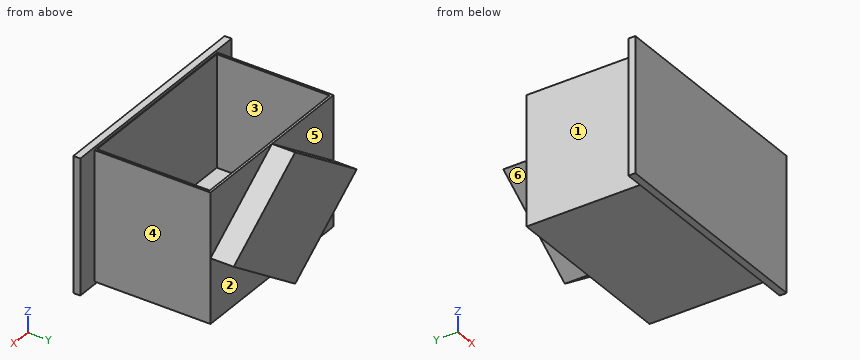
```python
from build123d import *

# Parameters (mm, degrees)
SKETCH_1_W          = 480
SKETCH_1_H          = 290
EXTRUDE_1_DEPTH     = 15
SKETCH_2_W          = 390
SKETCH_2_H          = 178
EXTRUDE_2_DEPTH     = 250
SKETCH_7_W          = 390
SKETCH_7_H          = 250
EXTRUDE_7_DEPTH     = 100
SKETCH_8_W          = 380
SKETCH_8_H          = 243
CUT_EXTRUDE_1_DEPTH = 240
EXTRUDE_8_DEPTH     = 50


with BuildPart() as part:
    # 草图1 → 凸台-拉伸1 (new body)
    with BuildSketch(Plane(origin=(0, 0, 0), x_dir=(1, 0, 0), z_dir=(0, 1, 0))):
        Rectangle(SKETCH_1_W, SKETCH_1_H)
    extrude(amount=-EXTRUDE_1_DEPTH)

    # 草图2 → 凸台-拉伸2 (add)
    with BuildSketch(Plane(origin=(0, 0, 0), x_dir=(1, 0, 0), z_dir=(0, 1, 0))):
        with Locations((0, 50)):
            Rectangle(SKETCH_2_W, SKETCH_2_H)
    extrude(amount=EXTRUDE_2_DEPTH)

    # 草图7 → 凸台-拉伸7 (add)
    with BuildSketch(Plane.XY.offset(39)):
        with Locations((0, 125)):
            Rectangle(SKETCH_7_W, SKETCH_7_H)
    extrude(amount=EXTRUDE_7_DEPTH)

    # 草图8 → 切除-拉伸1 (cut)
    with BuildSketch(Plane.XY.offset(139)):
        with Locations((0, 123.5)):
            Rectangle(SKETCH_8_W, SKETCH_8_H)
    extrude(amount=-CUT_EXTRUDE_1_DEPTH, mode=Mode.SUBTRACT)

    # 草图10 → 凸台-拉伸8 (add)
    with BuildSketch(Plane(origin=(0, 250, 0), x_dir=(1, 0, 0), z_dir=(0, 1, 0))):
        Polygon((0, 139), (-195, 0), (0, -139), (195, 0), align=None)
    extrude(amount=EXTRUDE_8_DEPTH)


solid = part.part
```
Input: part model. Units: mm. Frame: model coordinates. Face numbers are marked on the shaded views. A direction names the side the tool comes from. Coordinates: 2 decimals unless noted, no trailing zeros. Loops run counter-clockwise (first coordinate to the right, second up) from the corner with the lowest first, then second, coordinate; pieces in that order, holes last. Notation, with made-up numbers: M 0.25,77 L 18.25,77 A19 cw 18.25,87 Z; hole C 30.25,-32 d2. An arc over 180 degrees is marked long. One line per item, written item: value.
(1) Reachability of the marked faces 4, 5 and 6 from +Z, -Z, +X, -X, +Y, -Y: full face, straight path, thin tool, end or side. Return the list, or none.
Filled in:
face 4: +Z, -Z, +X, +Y
face 5: +Z, -X, +Y
face 6: -Z, -X, +Y
(2) Section B-B (x = -168.5). Output: boundary loops of the cut face in (y, z), and give its area (3 significant figures).
Filled in:
outline: M -15,-145 L 0,-145 L 0,-139 L 250,-139 L 250,-18.89 L 300,-18.89 L 300,18.89 L 250,18.89 L 250,139 L 245,139 L 245,-101 L 2,-101 L 2,139 L 0,139 L 0,145 L -15,145 Z
area: 17,400 mm^2
(3) Pin query (flat end, axial travel): pin 1 (2 mm diameter, centred on x = 122, z = 81.5, fed in from +Y); pin 2 (10 mm diameter, centred on y = 28, z = -23.5, fed in from +X); pin 3 (1.5 mm diameter, centred on y = 64.5, z = 111, fed in from -X). Return the tip coordinate at first contact, or that it passes through.
Filled in:
pin 1: y = 250
pin 2: x = 195
pin 3: x = -195
(4) Line query: line 1 along X through (y, z) = (45, 15); line 2 along Y through (x, z) = (-120.5, -28.5); line 3 along Y through (x, z) = (175, -40). Output: solid intervals per line, ascending. Write a range as from..to.
Filled in:
line 1: -195..-190, 190..195
line 2: -15..2, 245..300
line 3: -15..2, 245..250
(5) Section C-C (y = 12.5). Output: boundary loops of the cut face in (x, z), and give its area (3 significant figures).
Filled in:
outline: M -195,-139 L 195,-139 L 195,139 L 190,139 L 190,-101 L -190,-101 L -190,139 L -195,139 Z
area: 17,200 mm^2
(6) Section D-D (z = -110.5). Output: boundary loops of the cut face in (x, y), and give its area (3 significant figures).
Filled in:
outline: M -240,-15 L 240,-15 L 240,0 L 195,0 L 195,250 L 39.98,250 L 39.98,300 L -39.98,300 L -39.98,250 L -195,250 L -195,0 L -240,0 Z
area: 109,000 mm^2
(7) Pull-direction query (X, two-part tool) for the marked faces 1, 2 and 3; classes: +X half, -X half, draft (parallel to the pull), parting line (faces both ways), or undercut.
Filled in:
face 1: -X half
face 2: draft
face 3: undercut
(8) Section A-A (z = -6). Output: boundary loops of the cut face in (x, y), and give its area (3 significant figures).
Filled in:
outline: M -240,-15 L 240,-15 L 240,0 L 195,0 L 195,250 L 186.58,250 L 186.58,300 L -186.58,300 L -186.58,250 L -195,250 L -195,0 L -240,0 Z; hole M -190,2 L 190,2 L 190,245 L -190,245 Z
area: 31,000 mm^2
